Autodesk Inventor part; units mm, degrees
ref_plane "YZ Plane" through (0, 0, 0) normal (1, 0, 0) x (0, 1, 0)
ref_plane "XZ Plane" through (0, 0, 0) normal (0, 1, 0) x (-1, 0, 0)
ref_plane "XY Plane" through (0, 0, 0) normal (0, 0, 1) x (1, 0, 0)
sketch "Sketch1" plane through (0, 0, 0) normal (0, 0, 1) x (1, 0, 0)
  line L0 (0, 0) -> (16, 0)
  line L1 (16, 0) -> (16, 10)
  line L2 (16, 10) -> (0, 10)
  line L3 (0, 10) -> (0, 0)
  dimension "d0" = 16
  dimension "d1" = 10
extrude "Extrusion1" add sketch "Sketch1" along normal blind 3
sketch "Sketch2" plane through (0, 0, 3) normal (0, 0, 1) x (1, 0, 0)
  line L0 (1, 1) -> (15, 1)
  line L1 (15, 1) -> (15, 9)
  line L2 (15, 9) -> (1, 9)
  line L3 (1, 9) -> (1, 1)
  dimension "d4" = 14
  dimension "d5" = 8
extrude "Extrusion2" cut sketch "Sketch2" against normal through all
sketch "Sketch3" plane through (0, 10, 0) normal (0, 1, 0) x (1, 0, 0)
  line L0 (0, -3) -> (16, -3)
  line L1 (16, 0) -> (0, 0)
  line L2 (0, 0) -> (0, -3)
  line L3 (6, -3) -> (10, -3)
  line L4 (10, -3) -> (10, 0)
  line L5 (10, 0) -> (6, 0)
  line L6 (6, 0) -> (6, -3)
  dimension "d13" = 4
  dimension "d14" = 6
extrude "Extrusion3" add sketch "Sketch3" along normal blind 4 contours L6 L1 L4 L0
sketch "Sketch6" plane through (0, 0, 3) normal (0, 0, 1) x (1, 0, 0)
  point P0 (8, 12)
hole "Hole1" at (8, 12, 3) direction (0, 0, -1) diameter 1.524 end through all
thread "Thread1"
sketch "Sketch7" plane through (0, 0, 0) normal (0, -1, 0) x (1, 0, 0)
  line L0 (0, 0) -> (0, 3)
  line L1 (0, 0) -> (16, 0)
  line L2 (7, 0) -> (9, 0)
  line L3 (9, 0) -> (9, 1)
  line L4 (9, 1) -> (7, 1)
  line L5 (7, 1) -> (7, 0)
  dimension "d29" = 2
  dimension "d30" = 1
  dimension "d31" = 7
extrude "Extrusion5" add sketch "Sketch7" along normal blind 1
fillet "Fillet2" radius 0.5 14 edges at (1, 9, 1.5) (15, 9, 1.5) (15, 1, 1.5) (1, 1, 1.5) (10, 10, 1.5) (6, 10, 1.5) (6, 14, 1.5) (10, 14, 1.5) (16, 10, 1.5) (16, 0, 1.5) (0, 0, 1.5) (0, 10, 1.5) (7, 0, 0.5) (9, 0, 0.5)
properties part number "base"
Here's how the part is built. I have some questions about the finished solid (model axes, mm). A direction names the side the tool comes from. Give positions to 0.01 mm unless a question says otherwise; leave off trailing zeros. Order: outer loops, then holes, each group sorted by start corner. A loop starts at its lowest first (then second) coordinate and runs counter-clockwise, first axis right, second up. Notation, with made-up numbers: (4, -22.5) -> (13, -22.5) arc R23 cw to (13, 13.5) -> close; hole circle Ø11 at (-28.5, 65.25). An arc over 180 degrees is marked (long way). One line per item, written item: value. Start each with the question number.
1. Imagine slicing it at B-B, the plane x = 8. List the corners of the cut face in (y, z) for me.
2. For faces 4 (the face through (8, -0.5, 1)), 5 (the face through (16, 5, 1)), 6 (the face through (13, 10, 1)), 7 (the face through (6, 12, 1)), 8 (the face through (8, 1, 2)), which set-ups out of +Z, -Z, +X, -X, +Y, -Y let a thin tool reach every point of the face, with its end or its side?
3. Imagine slicing it at A-A, the plane z = 0.25. Count the separate pieces of the cut face and the enclosed holes in it, plus the area to 3 significant figures.
4. Imagine slicing it at D-D, the plane x = 14.25. List the corners of the cut face in (y, z) for me, plus the area to 3 significant figures.
5. We'd pull the mould along X, two halves only. Please class faces 1 (the face through (8, 9, 2)), 2 (the face through (7.9, 0, 1.5)), 3 (the face through (10, 12, 2)): released by +X, released by -X, zero draft, split by the parting line, or undercut.
6. I need wall thicknesses on probe 1 along Y at (x, z) = (8, 1.5); probe 2 along Y at (x, z) = (8, 0.7); probe 3 along X at (y, z) = (5, 1.4). Which ranges of each line are inside material? Lowest first, please. Write a range as from..to.
7. Imagine slicing it at C-C, the plane y = 7.75. List the corners of the cut face in (x, z) for me, plus the area to 3 significant figures.
8. Will these pins go through, and if not, where does the flat tip stop? pin 1 Ø1.5 at (x, z) = (5, 1.5) entering from -Y; pin 2 Ø2.5 at (x, y) = (8, 12) entering from -Z.
Values follow:
1. outline: (-1, 0) -> (1, 0) -> (1, 3) -> (0, 3) -> (0, 1) -> (-1, 1) -> close; (9, 0) -> (11.24, 0) -> (11.24, 3) -> (9, 3) -> close; (12.76, 0) -> (14, 0) -> (14, 3) -> (12.76, 3) -> close
2. face 4: +Z, +X, -X, -Y
2. face 5: +Z, -Z, +X, +Y, -Y
2. face 6: +Z, -Z, +X, +Y
2. face 7: +Z, -Z, -X, +Y
2. face 8: +Z, -Z
3. separate pieces: 1
3. enclosed holes: 2
3. area: 64.3 mm2
4. outline: (0, 0) -> (1, 0) -> (1, 3) -> (0, 3) -> close; (9, 0) -> (10, 0) -> (10, 3) -> (9, 3) -> close
4. area: 6.00 mm2
5. face 1: undercut
5. face 2: zero draft
5. face 3: released by +X
6. probe 1: y = 0..1, 9..11.24, 12.76..14
6. probe 2: y = -1..1, 9..11.24, 12.76..14
6. probe 3: x = 0..1, 15..16
7. outline: (0, 0) -> (1, 0) -> (1, 3) -> (0, 3) -> close; (15, 0) -> (16, 0) -> (16, 3) -> (15, 3) -> close
7. area: 6.00 mm2
8. pin 1: stops at y = 0
8. pin 2: stops at z = 0
